Read the model definition and answer for the solid it produces. Units are mm, in the model's axes. A direction names the side the tool comes from. Coordinates: 2 decimals unless noted, no trailing zeros. Order: outer loops, then holes, each group sorted by start corner. A loop starts at its lowest first (then second) coordinate and runs counter-clockwise, first axis right, second up. Notation, with made-up numbers: (-32.5, -20) -> (-15.5, -20) arc R23 ccw to (-15.5, -8) -> close; hole circle Ø11 at (3, 48). An arc over 180 degrees is marked (long way). Use CSV: the item, a comma, the result in double quotes.
```python
from build123d import *

# Parameters (mm, degrees)
PAD_DEPTH    = 4.05
PAD001_DEPTH = 3.85
PAD002_DEPTH = 4.05
PAD003_DEPTH = 3.85
POCKET_DEPTH = 0.15


with BuildPart() as part:
    # MirroredSketch001 → Pad (new body, symmetric)
    with BuildSketch(Plane.XZ):
        Polygon((0, 0.2), (0, 3.5), (-3.85, 3.5), (-3.85, 1.75), (-1.894893, 1.75), (-1, 0.2), align=None)
    extrude(amount=PAD_DEPTH, both=True)

    # MirroredSketch → Pad001 (join, symmetric)
    with BuildSketch(Plane.YZ):
        Polygon((-2, 0.2), (-2.894893, 1.75), (-4.05, 1.75), (-4.05, 3.5), (0, 3.5), (0, 0.2), align=None)
    extrude(amount=PAD001_DEPTH, both=True)

    # Sketch001 → Pad002 (join, symmetric)
    with BuildSketch(Plane.XZ):
        Polygon((0, 0.2), (0, 3.5), (3.85, 3.5), (3.85, 1.75), (1.894893, 1.75), (1, 0.2), align=None)
    extrude(amount=PAD002_DEPTH, both=True)

    # Sketch → Pad003 (join, symmetric)
    with BuildSketch(Plane.YZ):
        Polygon((2, 0.2), (2.894893, 1.75), (4.05, 1.75), (4.05, 3.5), (0, 3.5), (0, 0.2), align=None)
    extrude(amount=PAD003_DEPTH, both=True)

    # Sketch002 (on Face20 of Pad003) → Pocket (cut)
    with BuildSketch(Plane.XY.offset(3.5)):
        Polygon((-0.4, 2.8), (3.2, 2.8), (3.2, -0.8), (0.78, -0.8), (-0.4, 0.38), align=None)
    extrude(amount=-POCKET_DEPTH, mode=Mode.SUBTRACT)


solid = part.part
```
Item 1: Find section D-D, the plane z = 0.7. Give the vertices of the cut face in (x, y), then the cut area to 3 significant figures.
Return value:
outline,"(-3.85, -2.29) -> (-1.29, -2.29) -> (-1.29, -4.05) -> (1.29, -4.05) -> (1.29, -2.29) -> (3.85, -2.29) -> (3.85, 2.29) -> (1.29, 2.29) -> (1.29, 4.05) -> (-1.29, 4.05) -> (-1.29, 2.29) -> (-3.85, 2.29) -> close"
area,"44.3 mm^2"
Item 2: The mould has two halves that part along X. Classify faces 5 (the flat face through (-2.72, 2.44, 0.96)), 6 (the flat face through (1, 1, 3.35)), 7 (the flat face through (-1.454, 3.238, 0.986)), 8 (the flat face through (1.454, 3.238, 0.986)): +X half, -X half, draft (parallel to the pull), parting line (faces both ways), or undercut.
Return value:
face 5,"draft"
face 6,"undercut"
face 7,"-X half"
face 8,"+X half"
Item 3: Find section A-A, the plane x = 3. Give the vertices of the cut face in (y, z).
Return value:
outline,"(-4.05, 1.75) -> (-2.89, 1.75) -> (-2, 0.2) -> (2, 0.2) -> (2.89, 1.75) -> (4.05, 1.75) -> (4.05, 3.5) -> (2.8, 3.5) -> (2.8, 3.35) -> (-0.8, 3.35) -> (-0.8, 3.5) -> (-4.05, 3.5) -> close"
Item 4: Find section B-B, the plane y = 0.25. Give the vertices of the cut face in (x, z), then the cut area to 3 significant figures.
Return value:
outline,"(-3.85, 0.2) -> (3.85, 0.2) -> (3.85, 3.5) -> (3.2, 3.5) -> (3.2, 3.35) -> (-0.27, 3.35) -> (-0.27, 3.5) -> (-3.85, 3.5) -> close"
area,"24.9 mm^2"
Item 5: A tool of negligible diameter and unlimited length cuts with its end or side. For faces 1 (the flat face through (2.76, 2.44, 0.96)), 2 (the flat face through (-2.9, 3.5, 1.75)), 3 (the flat face through (-2.9, -3.5, 1.75)), 4 (the flat face through (2.76, -2.44, 0.96)), from which of +Z, -Z, +X, -X, +Y, -Y can it reach the whole face along a straight path? Write none if from no direction.
Return value:
face 1,"-Z, +X, +Y"
face 2,"-Z, -X, +Y"
face 3,"-Z, -X, -Y"
face 4,"-Z, +X, -Y"
Item 6: Straight lines are drawn through the part: line 1 along Z through (x, y) = (1, 0.75); line 2 along Z through (x, y) = (3.5, 3.5); line 3 along Y through (x, z) = (2, 1.5). For each, find the intervals that lie inside material, in ascending order.
Return value:
line 1,"z = 0.2 to 3.35"
line 2,"z = 1.75 to 3.5"
line 3,"y = -2.75 to 2.75"
Item 7: Find section C-C, the plane x = 0.25. Give the vertices of the cut face in (y, z), then the cut area to 3 significant figures.
Return value:
outline,"(-4.05, 0.2) -> (4.05, 0.2) -> (4.05, 3.5) -> (2.8, 3.5) -> (2.8, 3.35) -> (-0.27, 3.35) -> (-0.27, 3.5) -> (-4.05, 3.5) -> close"
area,"26.3 mm^2"
Item 8: Each of these flat-tipped pins is pushed along its axis until it touches: P1, Ø0.6, axis at x = 3, y = 3.5, coming from the -Z side; P2, Ø1, axis at x = 2.5, y = 2.5, coming from the +Z side; P3, Ø1.3, axis at x = -3.5, y = -3.5, coming from the -Z side; P4, Ø1.1, axis at x = 0.5, y = 1, coming from the +Z side. Where does it stop, or does it pass through?
Return value:
P1,"stops at z = 1.75"
P2,"stops at z = 3.5"
P3,"stops at z = 1.67"
P4,"stops at z = 3.35"
